Verification items for the finished model (mm, model axes). Face numbers are marked on the shaded views. A direction names the side the tool comes from. Give positions to 0.01 mm unless a question says otherwise; leave off trailing zeros. Write each loop counter-clockwise with the first axis right and the second up, starting at its lowest first coordinate (ties: lowest second). Pieces come first, ordered by that corner, then holes.
from build123d import *

# Parameters (mm, degrees)
F0_W      = 29
F0_H      = 16.5
F1_DEPTH  = 38.5
F2_T      = -2
F3_DEPTH  = 2.25
F4_SIZE   = 2
F5_SIZE   = 2
F6_SIZE   = 1
F8_DEPTH  = 16.501
F9_W      = 7.54
F9_H      = 7.25
F9_R      = 1.1
F10_DEPTH = 6.35
F11_W     = 5.398
F11_H     = 5.533
F13_W     = 5.538
F13_H     = 4.583


with BuildPart() as f1:
    # F0 (on Top) → F1 (new body)
    with BuildSketch(Plane.XY):
        with Locations((14.5, 8.25)):
            Rectangle(F0_W, F0_H)
    extrude(amount=F1_DEPTH)

    # F2
    f2_openings = [f1.faces().sort_by_distance(p)[0] for p in [
        (14.5, 8.25, 38.5),
    ]]
    offset(amount=F2_T, openings=f2_openings)

    # F3 (add): a face of the model
    f3_faces = [f1.faces().sort_by_distance(p)[0] for p in [
        (14.5, 8.25, 2),
    ]]
    extrude(f3_faces, amount=F3_DEPTH)

    # F4
    f4_edges = [f1.edges().sort_by_distance(p)[0] for p in [
        (0, 0, 19.25),
        (0, 16.5, 19.25),
        (29, 16.5, 19.25),
        (29, 0, 19.25),
    ]]
    chamfer(f4_edges, length=F4_SIZE)

    # F5
    f5_edges = [f1.edges().sort_by_distance(p)[0] for p in [
        (0, 8.25, 0),
        (1, 15.5, 0),
        (1, 1, 0),
        (14.5, 16.5, 0),
        (14.5, 0, 0),
        (28, 15.5, 0),
        (28, 1, 0),
        (29, 8.25, 0),
    ]]
    chamfer(f5_edges, length=F5_SIZE)

    # F6
    f6_edges = [f1.edges().sort_by_distance(p)[0] for p in [
        (14.5, 0, 38.5),
        (28, 1, 38.5),
        (29, 8.25, 38.5),
        (28, 15.5, 38.5),
        (14.5, 16.5, 38.5),
        (1, 15.5, 38.5),
        (0, 8.25, 38.5),
        (1, 1, 38.5),
    ]]
    chamfer(f6_edges, length=F6_SIZE)

    # F7 (on face) → F8 (cut, through all)
    with BuildSketch(Plane(origin=(0, 16.5, 0), x_dir=(-1, 0, 0), z_dir=(0, 1, 0))):
        Polygon((-23.536, 8.664), (-23.536, 4.94), (-6.464, 4.94), (-6.464, 8.664), (-12.635, 12.834), (-17.365, 12.834), align=None)
    extrude(amount=-F8_DEPTH, mode=Mode.SUBTRACT)

    # F9 (on Right) → F10 (join)
    with BuildSketch(Plane.YZ):
        with Locations((8.25, 7.875)):
            Rectangle(F9_W, F9_H)
        with Locations((8.25, 9)):
            Circle(F9_R, mode=Mode.SUBTRACT)
    extrude(amount=F10_DEPTH)

    # F11 (on Right) → F14 section 0
    with BuildSketch(Plane.YZ):
        with Locations((8.32, 8.0385)):
            Rectangle(F11_W, F11_H)
    # F13 (on offset) → F14 section 1
    with BuildSketch(Plane(origin=(4.45, 0, 0), x_dir=(0, -1, 0), z_dir=(-1, 0, 0))):
        with Locations((-8.25, 8.5135)):
            Rectangle(F13_W, F13_H)
    loft(mode=Mode.SUBTRACT)


solid = f1.part
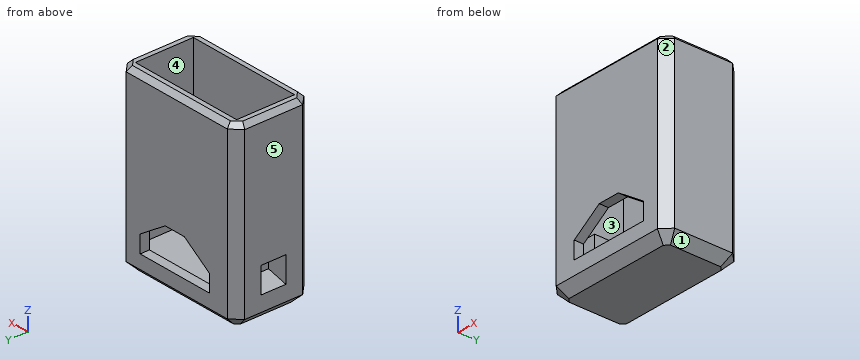
Item 1: Sectioned sample at C-C on y = 4. Record the cut outline in (x, z).
Answer key:
outline: (0, 2) - (2, 0) - (27, 0) - (29, 2) - (29, 37.5) - (28, 38.5) - (27, 38.5) - (27, 4.25) - (2, 4.25) - (2, 38.5) - (1, 38.5) - (0, 37.5) - close
Item 2: Set-up check for the marked faces 4 and 5: record each of +Z, -Z, +X, -X, +Y, -Y from which the full face is reachable in a straight line by a thin tool's end or side.
Answer key:
face 4: +Z
face 5: +Z, -Z, -X, +Y, -Y
Item 3: Depth check by flat-ended pin: pin 1 (2 mm diameter, centred on x = 4, y = 7, fed in from +Z); pin 2 (2.5 mm diameter, centred on y = 8, z = 9, fed in from -X); pin 3 (1.6 mm diameter, centred on y = 16, z = 7.5, fed in from -X). Enter the tip coordinate at first touch or a pass-through.
Answer key:
pin 1: stops at z = 11.5
pin 2: stops at x = 4.45
pin 3: stops at x = 0.7
Item 4: Sectioned sample at A-A on x = 23. Record the cut outline in (y, z).
Answer key:
outline: (0, 2) - (2, 0) - (14.5, 0) - (16.5, 2) - (16.5, 4.94) - (14.5, 4.94) - (14.5, 4.25) - (2, 4.25) - (2, 4.94) - (0, 4.94) - close; (0, 9.03) - (2, 9.03) - (2, 38.5) - (1, 38.5) - (0, 37.5) - close; (14.5, 9.03) - (16.5, 9.03) - (16.5, 37.5) - (15.5, 38.5) - (14.5, 38.5) - close
Item 5: Sectioned sample at B-B on z = 18. Record the cut outline in (x, y), then the cut area to 3 significant figures.
Answer key:
outline: (0, 2) - (2, 0) - (27, 0) - (29, 2) - (29, 14.5) - (27, 16.5) - (2, 16.5) - (0, 14.5) - close; hole (2, 2) - (27, 2) - (27, 14.5) - (2, 14.5) - close
area: 158 mm2
Item 6: Scan lines: line 1 along Y through (x, z) = (5.35, 9); line 2 along X through (y, z) = (14, 33); line 3 along Y through (x, z) = (24.25, 28). Record each from-to range of solid material in increasing order.
Answer key:
line 1: y = 0 to 2, 4.48 to 7.15, 9.35 to 12.02, 14.5 to 16.5
line 2: x = 0 to 2, 27 to 29
line 3: y = 0 to 2, 14.5 to 16.5
Item 7: Sectioned sample at D-D on z = 12. Record the cut outline in (x, y), then the cut area to 3 significant figures.
Answer key:
outline: (0, 2) - (2, 0) - (11.4, 0) - (11.4, 2) - (2, 2) - (2, 14.5) - (11.4, 14.5) - (11.4, 16.5) - (2, 16.5) - (0, 14.5) - close; (18.6, 0) - (27, 0) - (29, 2) - (29, 14.5) - (27, 16.5) - (18.6, 16.5) - (18.6, 14.5) - (27, 14.5) - (27, 2) - (18.6, 2) - close
area: 129 mm2
Item 8: Release check for a two-part mould opening along Y. For the marked faces 1, 2 and 3 record: released by +Y, released by -Y, zero draft, split by the parting line, or undercut.
Answer key:
face 1: zero draft
face 2: released by -Y
face 3: undercut
